Geometry check sheet. Reference: drawing and pictorial views, mm from the part's lowest x, y, z. Give positions to 0.01 mm unless a question says otherwise; leave off trailing zeros. Loops run counter-clockwise (first coordinate to the right, second up) from the corner with the lowest first, then second, coordinate; pieces in that order, holes last. Notation, with made-up numbers: (82, 58.25) -> (92, 58.25) arc R28 cw to (92, 87.25) -> close; hole circle Ø11 at (49, -13.5). An arc over 180 degrees is marked (long way). One line per item, written item: value. Start each with the question number.
(1) Sectioned sample at D-D, the plane z = 213. Record the cut outline in (x, y), then the cut area to 3 significant figures.
(2) Gauge pin test, flat ends, axial feed: pin 1 Ø4 at (x, y) = (120, 14) entering from -Z; pin 2 Ø0.9 at (x, z) = (19.5, 19.5) entering from -Y; pin 3 Ø1.5 at (x, y) = (70, 14.5) entering from -Z. Record the tip position at first contact, or that the pin passes through.
(3) Draft check along X on the marked faces 1, 2 and 3. Enter one of: pulls with the +X half, pulls with the -X half, needs draft (parallel to the pull), parting line crosses it, or undercut.
(4) Scan lines: line 1 along X through (y, z) = (3, 265); line 2 along Z through (x, y) = (20, 3); line 3 along X through (y, z) = (1.4, 20). Record each from-to range of solid material in increasing order. Write a range as from..to.
(5) Sectioned sample at C-C, the plane x = 46.5. Record the cut outline in (y, z), then the cut area to 3 significant figures.
(6) Sectioned sample at B-B, the plane y = 21. Record the cut outline in (x, z).
(7) Sectioned sample at A-A, the plane z = 63.5. Record the cut outline in (x, y), then the cut area to 3 significant figures.
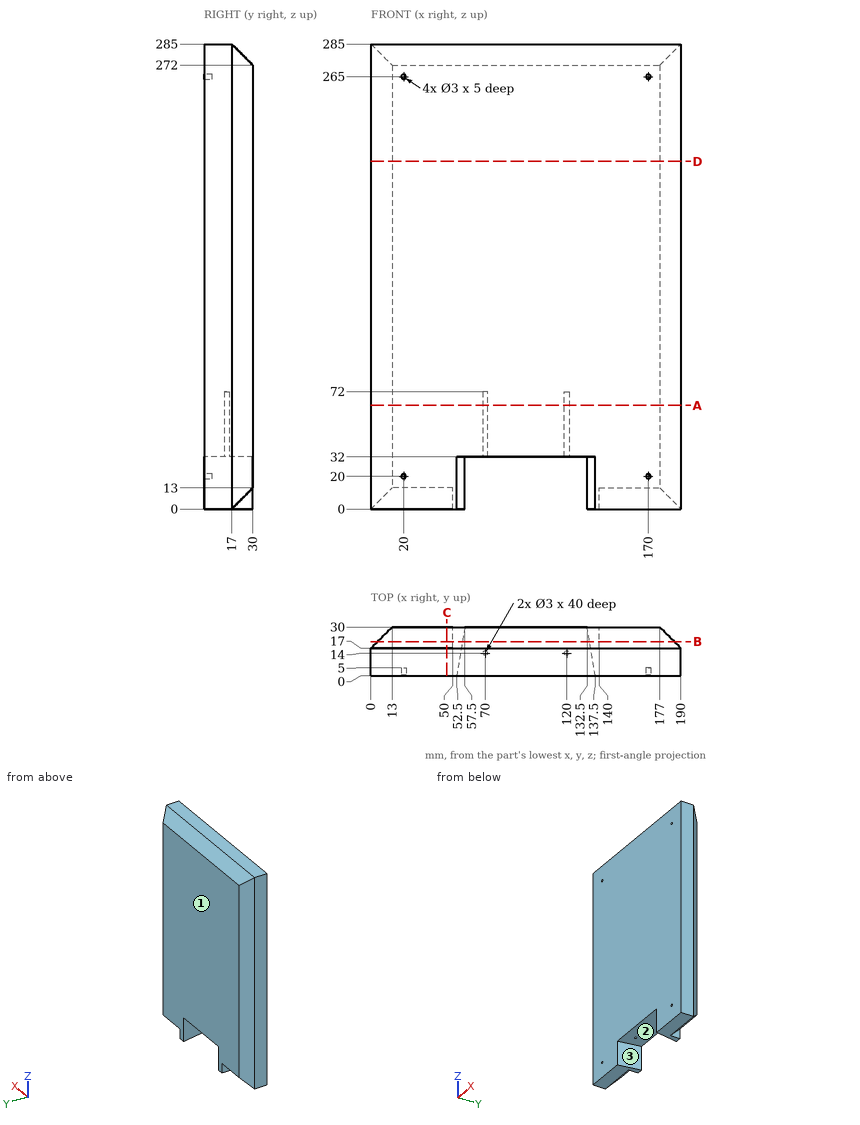
Calculated:
1. outline: (0, 0) -> (190, 0) -> (190, 17) -> (177, 30) -> (13, 30) -> (0, 17) -> close
1. area: 5,530 mm2
2. pin 1: stops at z = 32
2. pin 2: stops at y = 5
2. pin 3: stops at z = 72
3. face 1: needs draft
3. face 2: undercut
3. face 3: undercut
4. line 1: x = 0..18.5, 21.5..168.5, 171.5..190
4. line 2: z = 0..18.5, 21.5..263.5, 266.5..285
4. line 3: x = 0..18.5, 21.5..52.73, 137.27..168.5, 171.5..190
5. outline: (0, 0) -> (17, 0) -> (30, 13) -> (30, 272) -> (17, 285) -> (0, 285) -> close
5. area: 8,380 mm2
6. outline: (4, 4) -> (50, 4) -> (50, 0) -> (56, 0) -> (56, 32) -> (134, 32) -> (134, 0) -> (140, 0) -> (140, 4) -> (186, 4) -> (186, 281) -> (4, 281) -> close
7. outline: (0, 0) -> (190, 0) -> (190, 17) -> (177, 30) -> (13, 30) -> (0, 17) -> close; hole circle Ø3 at (70, 14); hole circle Ø3 at (120, 14)
7. area: 5,520 mm2
